```python
from build123d import *

# Parameters (mm, degrees)
F1_DEPTH = 2.54


with BuildPart() as f1:
    # F0 (on Top) → F1 (new body)
    with BuildSketch(Plane.XY):
        Polygon((-5.995896, -7.13228), (-6.844743, -6.480798), (-3.836085, 6.000167), (1.180427, 8.666), (7.587111, 8.666), (8.813967, 7.821221), (1.488084, 7.821221), (-1.447063, 6.26145), (6.127988, 6.26145), (5.180136, 2.561404), (10.624545, 2.561404), (11.634617, 6.504334), (7.82159, 9.129876), (1.097838, 9.129876), (-3.096944, 6.90072), (-0.511983, 16.991402), (-7.943114, 16.991402), (-6.19218, 15.589118), (-9.854238, 1.293863), (-14.809527, 1.293863), (-10.788241, 16.991402), (-18.210795, 16.991402), (-16.678699, 15.764381), (-20.272369, 1.022546), (-16.425734, -1.626137), (-9.515389, -1.626137), (-5.70774, 0.457038), (-7.423887, -6.662141), (-3.788898, -9.398828), (3.305492, -9.398828), (6.472039, -7.676311), (3.811726, -18.712221), (9.321281, -18.712221), (11.333264, -10.365812), (18.418461, -10.365812), (19.109229, -7.500265), (12.078154, -7.500265), (12.634992, -5.190304), (9.977397, -3.021413), (22.809136, -3.021413), (23.509286, -0.116946), (6.530533, -0.116946), (8.472281, -1.761667), (8.616393, -1.173794), (7.928506, -0.700135), (22.899743, -0.700135), (22.701854, -1.52105), (9.492916, -1.52105), (5.462863, -18.23912), (4.432984, -18.23912), (8.453434, -1.83855), (4.198023, -1.83855), (3.007288, -6.486717), (-2.007372, -6.486717), (0.705341, 4.102662), (-1.752948, 6.098899), (-2.961167, 5.456838), align=None)
        Polygon((-1.893178, -7.869553), (-1.667288, -6.998886), (3.390135, -6.998886), (4.516308, -2.327129), (7.205165, -2.327129), (6.993239, -3.206271), (5.234903, -3.206271), (4.110773, -7.869553), align=None, mode=Mode.SUBTRACT)
        Polygon((12.062723, -8.862222), (12.301775, -7.946932), (18.437441, -7.946932), (18.216802, -8.862222), align=None, mode=Mode.SUBTRACT)
        Polygon((-18.89434, 0.720949), (-19.655613, 1.344398), (-16.097893, 15.938756), (-16.728074, 16.443454), (-11.468086, 16.443454), (-11.679474, 15.576306), (-15.272995, 15.576306), align=None, mode=Mode.SUBTRACT)
        Polygon((-14.482171, 0.81359), (-9.49441, 0.81359), (-5.643328, 15.846721), (-6.503054, 16.535256), (-1.127594, 16.535256), (-1.376828, 15.562343), (-4.912582, 15.562343), (-8.926276, -0.105562), (-14.717633, -0.105562), align=None, mode=Mode.SUBTRACT)
        Polygon((5.828837, 2.995504), (6.583156, 5.94395), (7.486715, 5.94395), (6.775963, 2.995504), align=None, mode=Mode.SUBTRACT)
        Polygon((-3.836085, 6.000167), (-6.844743, -6.480798), (-5.995896, -7.13228), (-2.961167, 5.456838), (-1.752948, 6.098899), (-1.953123, 6.26145), (-1.447063, 6.26145), (1.488084, 7.821221), (8.813967, 7.821221), (7.587111, 8.666), (1.180427, 8.666), align=None)
        Polygon((-5.643328, 15.846721), (-9.49441, 0.81359), (-14.482171, 0.81359), (-14.717633, -0.105562), (-8.926276, -0.105562), (-4.912582, 15.562343), (-1.376828, 15.562343), (-1.127594, 16.535256), (-6.503054, 16.535256), align=None)
        Polygon((-16.097893, 15.938756), (-19.655613, 1.344398), (-18.89434, 0.720949), (-15.272995, 15.576306), (-11.679474, 15.576306), (-11.468086, 16.443454), (-16.728074, 16.443454), align=None)
        Polygon((7.486715, 5.94395), (6.583156, 5.94395), (5.828837, 2.995504), (6.775963, 2.995504), align=None)
        Polygon((8.563047, -1.83855), (8.453434, -1.83855), (4.432984, -18.23912), (5.462863, -18.23912), (9.492916, -1.52105), (22.701854, -1.52105), (22.899743, -0.700135), (7.928506, -0.700135), (8.616393, -1.173794), (8.472281, -1.761667), align=None)
        Polygon((3.390135, -6.998886), (-1.667288, -6.998886), (-1.893178, -7.869553), (4.110773, -7.869553), (5.234903, -3.206271), (6.993239, -3.206271), (7.205165, -2.327129), (4.516308, -2.327129), align=None)
        Polygon((18.437441, -7.946932), (12.301775, -7.946932), (12.062723, -8.862222), (18.216802, -8.862222), align=None)
    extrude(amount=F1_DEPTH)


solid = f1.part
```
Verification items for the finished model (mm, model axes). A direction names the side the tool comes from. Give positions to 0.01 mm unless a question says otherwise; leave off trailing zeros. Order: outer loops, then holes, each group sorted by start corner. A loop starts at its lowest first (then second) coordinate and runs counter-clockwise, first axis right, second up. Notation, with made-up numbers: M 69,51.25 L 94,51.25 A18 cw 94,70.25 Z; hole C 63.5,18 d6. An arc over 180 degrees is marked long. Return JSON: item names as keys, results as strings. Group by question number.
1) Section check D-D on y = -13. Record the cut outline in (x, z), and give its area (3 significant figures).
2) Section check A-A on y = 14.5. Record the cut outline in (x, z), and give its area (3 significant figures).
3) Go/stop test with flat-tipped pins: pin 1 Ø0.8 at (x, z) = (15.5, 1.5) entering from -Y; pin 2 Ø1.3 at (x, z) = (4, 0.5) entering from +Y; pin 3 Ø6 at (x, y) = (-2.5, -14.5) entering from -Z; pin 4 Ø6 at (x, y) = (-8.5, 11.5) entering from -Z. Record where each tip stops, or that it passes through.
4) Scan lines: line 1 (Y direction, x = 1.5, z = 2.05); line 2 (Y direction, x = 18, z = 2.3); line 3 (X direction, y = 6, z = 2.25). Record each from-to range of solid material in increasing order.
5) Section check B-B on y = 7.5. Record the cut outline in (x, z), and give its area (3 significant figures).
6) Mould release check, pull along Y, two halves, no side actions. Record for faces 6 (the face through (18.76, -8.95, 1.25)), 7 (the face through (11.3, -4.1, 1.3)), 8 (the face through (-2, 1, 0)): pulls with the +Y half, pulls with the -Y half, needs draft (parallel to the pull), parting line crosses it, or undercut.
7) Access from +Z, -Z, +X, -X, +Y, -Y to the whole of each face (thin tool, end or side, straight path). Record for faces 1 (the face through (7, -18.712, 1)), 2 (the face through (-13, -1.626, 1)), 3 (the face through (-12.827, 9.033, 1.252)), 4 (the face through (15, -0.117, 1)), 5 (the face through (-18.45, 8.5, 1.25)).
8) Section check C-C on x = -8.5. Record the cut outline in (y, z), and give its area (3 significant figures).
Answer block:
{
 "1": {"outline": "M 5.19,0 L 10.7,0 L 10.7,2.54 L 5.19,2.54 Z", "area": "14.0 mm^2"},
 "2": {"outline": "M -16.99,0 L -11.43,0 L -11.43,2.54 L -16.99,2.54 Z; M -6.47,0 L -1.15,0 L -1.15,2.54 L -6.47,2.54 Z", "area": "27.6 mm^2"},
 "3": {"pin 1": "stops at y = -10.37", "pin 2": "stops at y = 9.13", "pin 3": "passes through", "pin 4": "stops at z = 0"},
 "4": {"line 1": "y = -9.4 to -6.49, 6.26 to 9.13", "line 2": "y = -10.37 to -7.5, -3.02 to -0.12", "line 3": "x = -19.06 to -13.6, -8.65 to -1.63, 6.06 to 11.51"},
 "5": {"outline": "M -18.69,0 L -13.22,0 L -13.22,2.54 L -18.69,2.54 Z; M -8.26,0 L -2.94,0 L -2.94,2.54 L -8.26,2.54 Z; M -1.97,0 L 10.19,0 L 10.19,2.54 L -1.97,2.54 Z", "area": "58.3 mm^2"},
 "6": {"face 6": "pulls with the -Y half", "face 7": "undercut", "face 8": "needs draft"},
 "7": {"face 1": "+Z, -Z, +X, -X, -Y", "face 2": "+Z, -Z, -X, -Y", "face 3": "+Z, -Z", "face 4": "+Z, -Z, +X", "face 5": "+Z, -Z, -X"},
 "8": {"outline": "M -1.07,0 L 6.58,0 L 6.58,2.54 L -1.07,2.54 Z", "area": "19.4 mm^2"}
}
